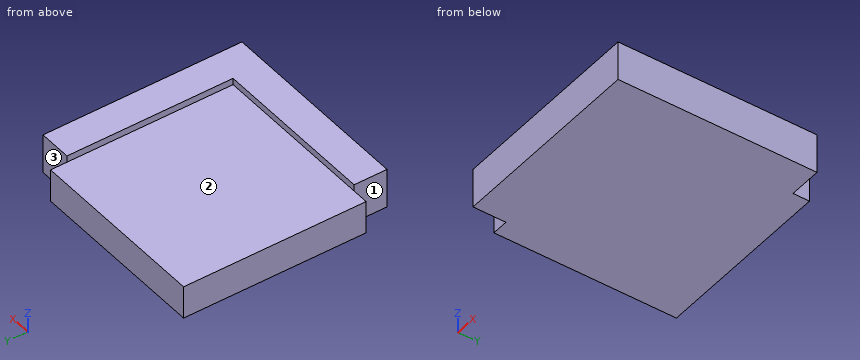
from build123d import *

# Parameters (mm, degrees)
F1_DEPTH = 12
F2_DEPTH = 10


with BuildPart() as f1:
    # F0 (on Top) → F1 (new body)
    with BuildSketch(Plane.XY):
        Polygon((-57.75, -20.25), (-90.75, -20.25), (-90.75, -30.25), (-30.25, -30.25), (-30.25, 30.25), (-40.25, 30.25), (-40.25, -2.5), (-40.25, -20.25), align=None)
    extrude(amount=F1_DEPTH)

    # F0 (on Top) → F2 (join)
    with BuildSketch(Plane.XY):
        Polygon((-90.75, -20.25), (-90.75, 30.25), (-40.25, 30.25), (-40.25, 35.2500006557), (-95.75, 35.2500006557), (-95.75, -20.25), align=None)
        Polygon((-40.25, 30.25), (-90.75, 30.25), (-90.75, -20.25), (-57.75, -20.25), (-40.25, -20.25), (-40.25, -2.5), align=None)
    extrude(amount=F2_DEPTH)


solid = f1.part
Part model, mm, in its own coordinate system. Face numbers are marked on the shaded views. A direction names the side the tool comes from. Coordinates: 2 decimals unless noted, no trailing zeros. Order: outer loops, then holes, each group sorted by start corner. A loop starts at its lowest first (then second) coordinate and runs counter-clockwise, first axis right, second up. Notation, with made-up numbers: M 89,-25 L 140,-25 A28 ccw 140,-1 Z; hole C 17.5,-9.75 d1. An arc over 180 degrees is marked long. Use a Markdown table: item, result.
(1) Cut at D-D on y = -26. Write the cut outline in (x, z), then the cut area to 3 significant figures.
A:
| item | result |
|---|---|
| outline | M -90.75,0 L -30.25,0 L -30.25,12 L -90.75,12 Z |
| area | 726 mm^2 |
(2) Tool access for the marked faces 1, 2 and 3: list every direction of +Z, -Z, +X, -X, +Y, -Y with a clear straight run to the whole face (end or side of a thin tool).
A:
| item | result |
|---|---|
| face 1 | +Z, -Z, -X, -Y |
| face 2 | +Z, -X, +Y |
| face 3 | +Z, -Z, +X, +Y |
(3) Cut at B-B on y = 0. Write the cut outline in (x, z), then the cut area to 3 significant figures.
A:
| item | result |
|---|---|
| outline | M -95.75,0 L -30.25,0 L -30.25,12 L -40.25,12 L -40.25,10 L -95.75,10 Z |
| area | 675 mm^2 |
(4) Cut at A-A on z = 3. Write the cut outline in (x, y), then the cut area to 3 significant figures.
A:
| item | result |
|---|---|
| outline | M -95.75,-20.25 L -90.75,-20.25 L -90.75,-30.25 L -30.25,-30.25 L -30.25,30.25 L -40.25,30.25 L -40.25,35.25 L -95.75,35.25 Z |
| area | 4,190 mm^2 |
(5) Probe L1, parallel to Z at x = -53, y = 2.5; L2, parallel to X at y = -25, z = 5; L3, parallel to Y at x = -33.5, z = 4. List the from-to ranges inside material, lowest first.
A:
| item | result |
|---|---|
| L1 | z = 0 to 10 |
| L2 | x = -90.75 to -30.25 |
| L3 | y = -30.25 to 30.25 |
(6) Cut at C-C on x = -76.5. Write the cut outline in (y, z), then the cut area to 3 significant figures.
A:
| item | result |
|---|---|
| outline | M -30.25,0 L 35.25,0 L 35.25,10 L -20.25,10 L -20.25,12 L -30.25,12 Z |
| area | 675 mm^2 |
(7) Flat gauge pins, fed straight in: pin 1 (4 mm diameter, centred on y = 32.5, z = 3.5, fed in from +X); pin 2 (1 mm diameter, centred on y = 14, z = 11, fed in from -X); pin 3 (4 mm diameter, centred on x = -94, z = 5.5, fed in from -Y). Where does each tip first touch, or does it go through?
A:
| item | result |
|---|---|
| pin 1 | stops at x = -40.25 |
| pin 2 | stops at x = -40.25 |
| pin 3 | stops at y = -20.25 |
